Job drawing, mm, ordinate dimensions from the low corner. One solid piece. Round coordinates to 2 decimals unless told otherwise and drop trailing zeros. Order: outer loops, then holes, each group sorted by start corner. A loop starts at its lowest first (then second) coordinate and runs counter-clockwise, first axis right, second up. Notation, with made-up numbers: (25, 11) -> (77, 11) arc R20 cw to (77, 18) -> close; hole circle Ø5 at (33.25, 0.25). An arc over 180 degrees is marked (long way). Return JSON: item names as keys, results as strings. Group by question number.
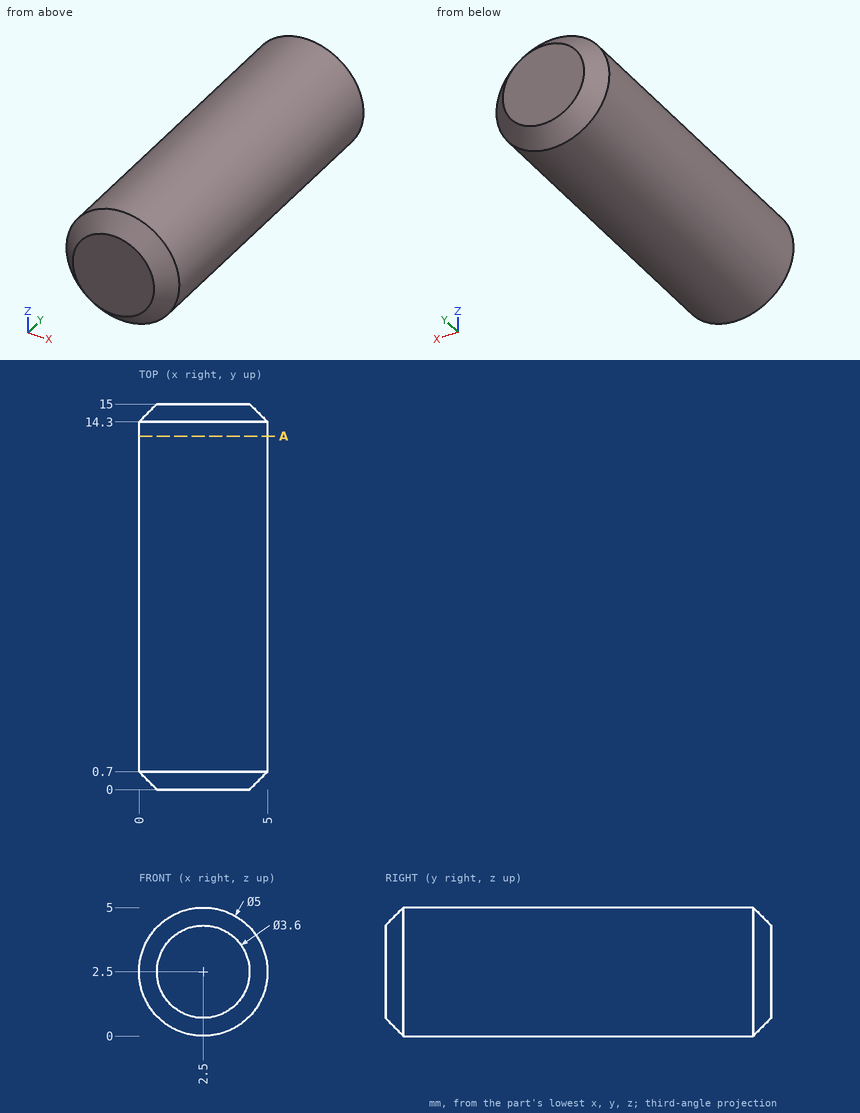
(1) Saw through at A-A, the plane y = 13.75. List the corners of the cut face in (x, z).
(2) Pin check, flat tip, straight feed: P1, Ø1, axis at y = 5.5, z = 1.5, coming from the +X side. Stop position of the tip, or through.
(3) Probe L1, parallel to X at y = 4.5, z = 4.7; L2, parallel to X at y = 11, z = 1; L3, parallel to Y at x = 0.4, z = 3.4. List the from-to ranges inside material, lowest first. Write a range as [from, to].
Results are:
{
 "1": {"outline": "circle Ø5 at (2.5, 2.5)"},
 "2": {"P1": "stops at x = 4.95"},
 "3": {"L1": "x = [1.31, 3.69]", "L2": "x = [0.5, 4.5]", "L3": "y = [0.48, 14.52]"}
}
